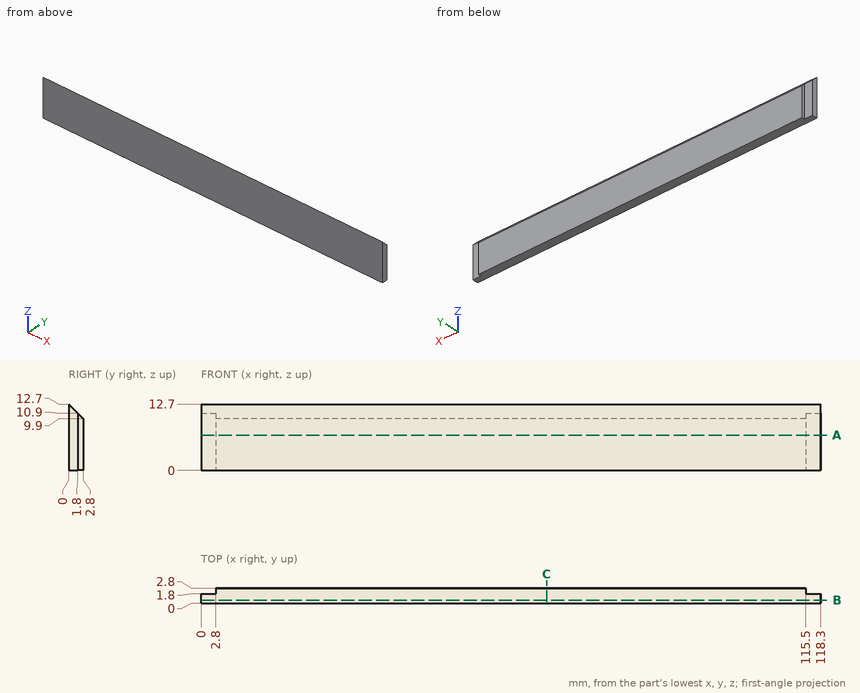
Study the drawing (mm; zero at the part's minimum x, y, z) and answer. Coordinates: 2 decimals unless noted, no trailing zeros. Write each loop counter-clockwise with the first axis right and the second up, starting at its lowest first coordinate (ties: lowest second). Pieces come first, ordered by that corner, then holes. Notation, with made-up numbers: (-17.5, 31.5) - (27.5, 31.5) arc R22 cw to (27.5, 39.5) - close; hole circle Ø9 at (57.5, 39). An arc over 180 degrees is marked (long way). Answer as a JSON object with one key per item and string values. Group by question number.
1. A cutting plane is placed at A-A (z = 6.75). Determine the outline of the cut face in (x, y).
2. A cutting plane is placed at C-C (x = 66). Determine the outline of the cut face in (y, z), plus the area to 3 significant figures.
3. This flat-tipped pin is pushed along its axis until it touches: P1, Ø1.4, axis at x = 1, z = 4.5, coming from the +Y side. Where does it stop, or does it pass through?
4. A cutting plane is placed at B-B (y = 0.6). Determine the outline of the cut face in (x, z).
5. Consider L1, parallel to X at y = 2.15, z = 5.5; L2, parallel to Z at x = 70, y = 0.65; L3, parallel to Z at x = 51.5, y = 2. Determine where each line is inside the solid, lowest interval first. Write a range as [from, to].
Worked out:
{
 "1": {"outline": "(0, 0) - (118.3, 0) - (118.3, 1.8) - (115.5, 1.8) - (115.5, 2.8) - (2.8, 2.8) - (2.8, 1.8) - (0, 1.8) - close"},
 "2": {"outline": "(0, 0) - (2.8, 0) - (2.8, 9.9) - (0, 12.7) - close", "area": "31.6 mm²"},
 "3": {"P1": "stops at y = 1.8"},
 "4": {"outline": "(0, 0) - (118.3, 0) - (118.3, 12.1) - (0, 12.1) - close"},
 "5": {"L1": "x = [2.8, 115.5]", "L2": "z = [0, 12.05]", "L3": "z = [0, 10.7]"}
}
